```python
from build123d import *

# Parameters (mm, degrees)
BOSS_EXTRUDE1_START = -80
BOSS_EXTRUDE1_DEPTH = 1.6
CHAMFER1_SIZE       = 0.5
BOSS_EXTRUDE2_START = -81
BOSS_EXTRUDE2_DEPTH = 3
CHAMFER2_SIZE       = 0.5
BOSS_EXTRUDE3_START = -81
BOSS_EXTRUDE3_DEPTH = 3
CHAMFER3_SIZE       = 0.5
BOSS_EXTRUDE4_START = -80.1
SKETCH4_W           = 3
SKETCH4_H           = 0.9
BOSS_EXTRUDE4_DEPTH = 0.9
BOSS_EXTRUDE5_START = -32
BOSS_EXTRUDE5_DEPTH = 4
BOSS_EXTRUDE6_START = 28
BOSS_EXTRUDE6_DEPTH = 4


with BuildPart() as part:
    # Sketch1 → Boss-Extrude1 (new body)
    with BuildSketch(Plane.XY.offset(BOSS_EXTRUDE1_START)):
        with BuildLine():
            Line((-32, 8.6), (32, 8.6))
            ThreePointArc((32, 8.6), (34.828427125, 9.771572875), (36, 12.6))
            Line((36, 12.6), (36, 30.6))
            ThreePointArc((36, 30.6), (34.828427125, 33.428427125), (32, 34.6))
            Line((32, 34.6), (-32, 34.6))
            ThreePointArc((-32, 34.6), (-34.828427125, 33.428427125), (-36, 30.6))
            Line((-36, 30.6), (-36, 12.6))
            ThreePointArc((-36, 12.6), (-34.828427125, 9.771572875), (-32, 8.6))
        make_face()
    extrude(amount=BOSS_EXTRUDE1_DEPTH)

    # Chamfer1
    chamfer1_edges = [part.edges().sort_by_distance(p)[0] for p in [
        (36, 21.6, -80),
        (34.828427125, 9.771572875, -80),
        (0, 8.6, -80),
        (-34.828427125, 9.771572875, -80),
        (-36, 21.6, -80),
        (-34.828427125, 33.428427125, -80),
        (0, 34.6, -80),
        (34.828427125, 33.428427125, -80),
    ]]
    chamfer(chamfer1_edges, length=CHAMFER1_SIZE)


with BuildPart() as body_2:
    # Sketch2 → Boss-Extrude2 (new body)
    with BuildSketch(Plane.XY.offset(BOSS_EXTRUDE2_START)):
        with BuildLine():
            Line((-3, 18.25), (3, 18.25))
            ThreePointArc((3, 18.25), (4.414213562, 18.835786438), (5, 20.25))
            Line((5, 20.25), (5, 24.25))
            ThreePointArc((5, 24.25), (4.414213562, 25.664213562), (3, 26.25))
            Line((3, 26.25), (-3, 26.25))
            ThreePointArc((-3, 26.25), (-4.414213562, 25.664213562), (-5, 24.25))
            Line((-5, 24.25), (-5, 20.25))
            ThreePointArc((-5, 20.25), (-4.414213562, 18.835786438), (-3, 18.25))
        make_face()
    extrude(amount=BOSS_EXTRUDE2_DEPTH)


with BuildPart() as part_1:
    add(part.part)

    # Combine1: cut body 2
    add(body_2.part, mode=Mode.SUBTRACT)

    # Chamfer2
    chamfer2_edges = [part_1.edges().sort_by_distance(p)[0] for p in [
        (-5, 22.25, -80),
        (-4.414213562, 25.664213562, -80),
        (0, 26.25, -80),
        (4.414213562, 25.664213562, -80),
        (5, 22.25, -80),
        (4.414213562, 18.835786438, -80),
        (0, 18.25, -80),
        (-4.414213562, 18.835786438, -80),
    ]]
    chamfer(chamfer2_edges, length=CHAMFER2_SIZE)


with BuildPart() as body_2_2:
    # Sketch3 → Boss-Extrude3 (new body)
    with BuildSketch(Plane.XY.offset(BOSS_EXTRUDE3_START)):
        with BuildLine():
            Line((24.5, 24.08), (30.5, 24.08))
            ThreePointArc((30.5, 24.08), (32.974873734, 25.105126266), (34, 27.58))
            ThreePointArc((34, 27.58), (32.974873734, 30.054873734), (30.5, 31.08))
            Line((30.5, 31.08), (24.5, 31.08))
            ThreePointArc((24.5, 31.08), (22.025126266, 30.054873734), (21, 27.58))
            ThreePointArc((21, 27.58), (22.025126266, 25.105126266), (24.5, 24.08))
        make_face()
    extrude(amount=BOSS_EXTRUDE3_DEPTH)


with BuildPart() as part_2:
    add(part_1.part)

    # Combine2: cut body 2 2
    add(body_2_2.part, mode=Mode.SUBTRACT)

    # Chamfer3
    chamfer3_edges = [part_2.edges().sort_by_distance(p)[0] for p in [
        (27.5, 31.08, -80),
        (34, 27.58, -80),
        (27.5, 24.08, -80),
        (21, 27.58, -80),
    ]]
    chamfer(chamfer3_edges, length=CHAMFER3_SIZE)


with BuildPart() as body_2_3:
    # Sketch4 → Boss-Extrude4 (new body)
    with BuildSketch(Plane.XY.offset(BOSS_EXTRUDE4_START)):
        with Locations((0, 8.95)):
            Rectangle(SKETCH4_W, SKETCH4_H)
    extrude(amount=BOSS_EXTRUDE4_DEPTH)


with BuildPart() as part_3:
    add(part_2.part)

    # Combine3: cut body 2 3
    add(body_2_3.part, mode=Mode.SUBTRACT)

    # Sketch5 → Boss-Extrude5 (add)
    with BuildSketch(Plane(origin=(0, 0, 0), x_dir=(0, 0, -1), z_dir=(1, 0, 0)).offset(BOSS_EXTRUDE5_START)):
        Polygon((78.41, 12), (74.6, 12), (74.6, 12.8), (74.9, 13.1), (75.2, 13.1), (75.2, 12.8), (78.41, 12.8), align=None)
    extrude(amount=BOSS_EXTRUDE5_DEPTH)

    # Sketch6 → Boss-Extrude6 (add)
    with BuildSketch(Plane(origin=(0, 0, 0), x_dir=(0, 0, -1), z_dir=(1, 0, 0)).offset(BOSS_EXTRUDE6_START)):
        Polygon((78.41, 12), (74.6, 12), (74.6, 12.8), (74.9, 13.1), (75.2, 13.1), (75.2, 12.8), (78.41, 12.8), align=None)
    extrude(amount=BOSS_EXTRUDE6_DEPTH)


solid = part_3.part
```
Build history of the part. All positions in model axes, mm. A direction names the side the tool comes from. Round coordinates to 2 decimals unless told otherwise and drop trailing zeros. Loops run counter-clockwise (first coordinate to the right, second up) from the corner with the lowest first, then second, coordinate; pieces in that order, holes last.
Item 1: Which spindle directions (+Z, -Z, +X, -X, +Y, -Y) get a long thin tool onto all of the face, cutting with end or side? Do faces 1 (the face through (30, 12, -77)), 2 (the face through (4.493, 25.776, -79.635)), 3 (the face through (-30, 12.8, -77)), 4 (the face through (-4.4, 25.68, -78.96)). Say none if no direction does.
Item 2: Saw through at C-C (y = 14.5). List the corners of the cut face in (x, z).
Item 3: Drill centre lines: line 1 along X through (y, z) = (23.25, -79); line 2 along Z through (x, y) = (-1, 31.5); line 3 along Y through (x, z) = (-20, -79.7). Where is each one in solid material? Low to high.
Item 4: Pin check, flat tips, straight feed: P1, Ø0.5, axis at y = 12.5, z = -76, coming from the -X side; P2, Ø0.6, axis at y = 9, z = -79.5, coming from the -X side; P3, Ø1.2, axis at y = 12.5, z = -77.5, coming from the +X side; P4, Ø2, axis at y = 18.5, z = -77.5, coming from the +X side. Stop position of each tip, or through.
Item 5: Two-plate mould, pull along X, no slides. Class faces 5 (the face through (0, 16, -80)), 6 (the face through (-34.859, 9.803, -78.958)), 7 (the face through (-4.526, 25.743, -79.635)), 8 (the face through (34.859, 33.397, -78.958)): released by +X, released by -X, zero draft, split by the parting line, or undercut.
Item 6: Saw through at B-B (x = -29). List the corners of the cut face in (y, z).
Item 7: Saw through at D-D (x = -7). List the corners of the cut face in (y, z), then the cut area to 4 significant figures.
Item 8: Saw through at A-A (z = -76.4). List the corners of the cut face in (x, y), then the cut area to 3 significant figures.
Worked answers:
1. face 1: +Z, +X, -X, -Y
1. face 2: -Z
1. face 3: +X, -X, +Y
1. face 4: +Z, -Z
2. outline: (-36, -79.5) - (-35.5, -80) - (35.5, -80) - (36, -79.5) - (36, -78.4) - (-36, -78.4) - close
3. line 1: x = -36 to -5, 5 to 36
3. line 2: z = -80 to -78.4
3. line 3: y = 8.8 to 34.4
4. P1: stops at x = -32
4. P2: stops at x = -34.26
4. P3: stops at x = 32
4. P4: stops at x = 36
5. face 5: zero draft
5. face 6: released by -X
5. face 7: undercut
5. face 8: released by +X
6. outline: (8.6, -79.5) - (9.1, -80) - (34.1, -80) - (34.6, -79.5) - (34.6, -78.4) - (12.8, -78.4) - (12.8, -75.2) - (13.1, -75.2) - (13.1, -74.9) - (12.8, -74.6) - (12, -74.6) - (12, -78.4) - (8.6, -78.4) - close
7. outline: (8.6, -79.5) - (9.1, -80) - (34.1, -80) - (34.6, -79.5) - (34.6, -78.4) - (8.6, -78.4) - close
7. area: 41.35 mm2
8. outline: (-32, 12) - (-28, 12) - (-28, 12.8) - (-32, 12.8) - close; (28, 12) - (32, 12) - (32, 12.8) - (28, 12.8) - close
8. area: 6.40 mm2
